from build123d import *

# Parameters (mm, degrees)
SKETCH1_W               = 2.7
SKETCH1_H               = 40
BOSS_EXTRUDE2_DEPTH     = 11
BOSS_EXTRUDE2_2_DEPTH   = 11
SKETCH3_W               = 25
SKETCH3_H               = 40
BOSS_EXTRUDE3_DEPTH     = 3
BOSS_EXTRUDE4_REACH     = 51.883
SKETCH4_W               = 40
SKETCH4_H               = 2
SKETCH5_W               = 30.4
SKETCH5_H               = 3
BOSS_EXTRUDE5_DEPTH     = 22.225
CUT_EXTRUDE1_DEPTH      = 70.714493651
CUT_EXTRUDE1_DEPTH_BACK = 70.714493651
SKETCH7_R               = 4.7625
CUT_EXTRUDE2_DEPTH      = 70.714493651
FILLET6_R               = 2
FILLET8_R               = 2
FILLET9_R               = 2
FILLET10_R              = 2


with BuildPart() as part:
    # Sketch1 → Boss-Extrude2 (new body)
    with BuildSketch(Plane(origin=(0, 0, 0), x_dir=(1, 0, 0), z_dir=(0, 1, 0))):
        with Locations((-29.05, 20)):
            Rectangle(SKETCH1_W, SKETCH1_H)
    extrude(amount=BOSS_EXTRUDE2_DEPTH)



with BuildPart() as body_2:
    # Sketch1 → Boss-Extrude2 2 (new body)
    with BuildSketch(Plane(origin=(0, 0, 0), x_dir=(1, 0, 0), z_dir=(0, 1, 0))):
        with Locations((-1.35, 20)):
            Rectangle(SKETCH1_W, SKETCH1_H)
    extrude(amount=BOSS_EXTRUDE2_2_DEPTH)


with BuildPart() as part_1:
    add(part.part)

    add(body_2.part)  # Boss-Extrude3 merges body 2
    # Sketch3 → Boss-Extrude3 (add)
    with BuildSketch(Plane(origin=(0, 0, 0), x_dir=(1, 0, 0), z_dir=(0, 1, 0))):
        with Locations((-15.2, 20)):
            Rectangle(SKETCH3_W, SKETCH3_H)
    extrude(amount=BOSS_EXTRUDE3_DEPTH)

    # Sketch4 → Boss-Extrude4 (add, up to next)
    with BuildSketch(Plane(origin=(-27.7, 0, 0), x_dir=(0, 0, -1), z_dir=(1, 0, 0)), mode=Mode.PRIVATE) as boss_extrude4_sk1:
        with Locations((20, 10)):
            Rectangle(SKETCH4_W, SKETCH4_H)
    boss_extrude4_tool1 = extrude(boss_extrude4_sk1.sketch, amount=BOSS_EXTRUDE4_REACH, mode=Mode.PRIVATE) - part_1.part
    add(boss_extrude4_tool1.solids().sort_by_distance((-27.7, 10, -20))[0])

    # Sketch5 → Boss-Extrude5 (add)
    with BuildSketch(Plane(origin=(0, 0, -40), x_dir=(-1, 0, 0), z_dir=(0, 0, -1))):
        with Locations((15.2, 1.5)):
            Rectangle(SKETCH5_W, SKETCH5_H)
    extrude(amount=BOSS_EXTRUDE5_DEPTH)

    # Sketch6 → Cut-Extrude1 (cut, two sides: drawn at the far end of the back side and taken through both)
    with BuildSketch(Plane(origin=(0, 3, 0), x_dir=(1, 0, 0), z_dir=(0, 1, 0)).offset(-CUT_EXTRUDE1_DEPTH_BACK)):
        with BuildLine():
            Line((33.516714256, -65.275403725), (0, 40))
            Line((0, 40), (-4.611193503, 54.483676829))
            ThreePointArc((-4.611193503, 54.483676829), (-15.153412609, 62.224902344), (-25.760168287, 54.572341326))
            Line((-25.760168287, 54.572341326), (-30.4, 40))
            Line((-30.4, 40), (-63.919403204, -65.274547602))
            Line((-63.919403204, -65.274547602), (-63.917461702, 155.689528782))
            Line((-63.917461702, 155.689528782), (33.518655758, 155.688672658))
            Line((33.518655758, 155.688672658), (33.516714256, -65.275403725))
        make_face()
    extrude(amount=CUT_EXTRUDE1_DEPTH + CUT_EXTRUDE1_DEPTH_BACK, mode=Mode.SUBTRACT)

    # Sketch7 → Cut-Extrude2 (cut, through all)
    with BuildSketch(Plane(origin=(0, 3, 0), x_dir=(1, 0, 0), z_dir=(0, 1, 0))):
        with Locations(Location((-15.176706304, 51.112451172, 0), (0, 0, 270))):
            Circle(SKETCH7_R)
    extrude(amount=-CUT_EXTRUDE2_DEPTH, mode=Mode.SUBTRACT)

    # Fillet6
    fillet6_edges = [part_1.edges().sort_by_distance(p)[0] for p in [
        (-15.2, 11, 0),
    ]]
    fillet(fillet6_edges, radius=FILLET6_R - 0.0001)  # a hair under: the kernel refuses the full size

    # Fillet8
    fillet8_edges = [part_1.edges().sort_by_distance(p)[0] for p in [
        (0, 4.50005, 0),
        (0, 10.414242852, -0.585757148),
        (-30.4, 4.50005, 0),
        (-30.4, 10.414242852, -0.585757148),
        (0, 11, -20.99995),
        (-30.4, 11, -20.99995),
    ]]
    fillet(fillet8_edges, radius=FILLET8_R - 0.0001)  # a hair under: the kernel refuses the full size

    # Fillet9
    fillet9_edges = [part_1.edges().sort_by_distance(p)[0] for p in [
        (0, 0, -20.99995),
        (-0.585757148, 0, -0.585757148),
        (-15.2, 0, 0),
        (-29.814242852, 0, -0.585757148),
        (-30.4, 0, -20.99995),
    ]]
    fillet(fillet9_edges, radius=FILLET9_R - 0.0001)  # a hair under: the kernel refuses the full size

    # Fillet10
    fillet10_edges = [part_1.edges().sort_by_distance(p)[0] for p in [
        (-1.35, 3, -40),
        (-29.05, 3, -40),
    ]]
    fillet(fillet10_edges, radius=FILLET10_R)


solid = part_1.part
Geometry: final body of the model. Coordinates: model frame, mm. A direction names the side the tool comes from. Coordinates: 2 decimals unless noted, no trailing zeros. Order: outer loops, then holes, each group sorted by start corner. A loop starts at its lowest first (then second) coordinate and runs counter-clockwise, first axis right, second up. Notation, with made-up numbers: M 48,18.5 L 74,18.5 A16 ccw 74,38.5 Z; hole C 80.25,31 d7. An arc over 180 degrees is marked long. One line per question, with ' | ' between items. Start each with the question number.
Item 1: Cut plane C-C, the plane x = -16. Count the separate pieces of the cut face and the enclosed holes in it, then the cut area to 3 significant figures.
Item 2: Pin query (flat end, axial travel): pin 1 Ø4 at (x, y) = (-14, 8.5) entering from -Z; pin 2 Ø15 at (x, z) = (-15.18, -51.11) entering from +Y; pin 3 Ø1 at (y, z) = (1.5, -38) entering from +X. Return the tip coordinate at first contact, or that it passes through.
Item 3: Cut plane A-A, the plane y = 5.75. Return the cut outline in (x, z), then the cut area to 3 significant figures.
Item 4: Set-up query: faces 1 (the flat face through (-2.7, 6, -21)), 2 (the flat face through (-2.273, 1.354, -47.14)). Return all of +Z, -Z, +X, -X, +Y, -Y with unobstructed straight access to the full face (end or side cutting, diameter ignored); none if empty.
Item 5: Ray query, probe 1 along Y at (x, z) = (-4, -6); probe 2 along X at (y, z) = (6.25, -32); probe 3 along Y at (x, z) = (-8, -42.5). Return the intervals inside material, ascending. Write a range as [from, to].
Item 6: Draft query along X for faces 3 (the flat face through (-15.4, 9.3, -40)), 4 (the flat face through (0, 5, -21)), 5 (the flat face through (-27.7, 6, -21)). Return one class per face: released by +X, released by -X, zero draft, split by the parting line, or undercut.
Item 7: Cut plane B-B, the plane z = -34. Return the cut outline in (x, y), then the cut area to 3 significant figures.
A:
1) separate pieces: 3 | enclosed holes: 0 | area: 237 mm2
2) pin 1: stops at z = -40 | pin 2: stops at y = 3 | pin 3: stops at x = 0
3) outline: M -30.4,-40 L -27.7,-40 L -27.7,0 L -28.4,0 A2 ccw -30.4,-2 Z; M -2.7,-40 L 0,-40 L 0,-2 A2 ccw -2,0 L -2.7,0 Z | area: 214 mm2
4) face 1: +Z, -Z | face 2: -Z, +X, +Y, -Y
5) probe 1: y = [0, 3], [9, 11] | probe 2: x = [-30.4, -27.7], [-2.7, 0] | probe 3: y = [0, 3]
6) face 3: zero draft | face 4: released by +X | face 5: undercut
7) outline: M -30.4,2 A2 ccw -28.4,0 L -2,0 A2 ccw 0,2 L 0,9 A2 ccw -2,11 L -28.4,11 A2 ccw -30.4,9 Z; hole M -27.7,3 L -2.7,3 L -2.7,9 L -27.7,9 Z | area: 181 mm2
